from build123d import *

# Parameters (mm, degrees)
REVOLVE_3_ANGLE               = 210
SKETCH_11_W                   = 1123.766968822
SKETCH_11_H                   = 50
CUT_REVOLVE_6_ANGLE           = 5
CUT_REVOLVE_6_OTHER_WAY_ANGLE = 180


with BuildPart() as part:
    # 草图4 → 旋转3 (revolve)
    with BuildSketch(Plane.XY):
        Polygon((-949.526197638, 0), (-949.526197638, -80), (-700, -80), (-700, 80), (-949.526197638, 80), align=None)
    revolve(axis=Axis((0, 0, 0), (0, 1, 0)), revolution_arc=REVOLVE_3_ANGLE)

    # 草图10 → 切除-旋转5 (revolve, cut)
    with BuildSketch(Plane(origin=(0, 0, 0), x_dir=(0.9659258262890681, 0, -0.2588190451025215), z_dir=(0.2588190451025215, 0, 0.9659258262890681)), mode=Mode.PRIVATE) as cut_revolve_5_sk:
        with BuildLine():
            Line((-750, 50), (750, 50))
            ThreePointArc((750, 50), (785.355339059, 35.355339059), (800, 0))
            Line((800, 0), (-800, 0))
            ThreePointArc((-800, 0), (-785.355339059, 35.355339059), (-750, 50))
        make_face()
    revolve(cut_revolve_5_sk.sketch.rotate(Axis((-1280.947086283, 0, 343.228737317), (0.9659258262890681, 0, -0.25881904510252157)), 90), axis=Axis((-1280.947086283, 0, 343.228737317), (0.9659258262890681, 0, -0.25881904510252157)), mode=Mode.SUBTRACT)

    # 草图11 → 切除-旋转6 (revolve, cut)
    with BuildSketch(Plane(origin=(0, 0, 0), x_dir=(0.9659258262890681, 0, -0.2588190451025215), z_dir=(0.2588190451025215, 0, 0.9659258262890681))):
        with Locations((-561.883484411, 0)):
            Rectangle(SKETCH_11_W, SKETCH_11_H)
    revolve(axis=Axis((0, 25, 0), (0, -1, 0)), revolution_arc=CUT_REVOLVE_6_ANGLE, mode=Mode.SUBTRACT)

    # 草图11 → 切除-旋转6 other way (revolve, cut)
    with BuildSketch(Plane(origin=(0, 0, 0), x_dir=(0.9659258262890681, 0, -0.2588190451025215), z_dir=(0.2588190451025215, 0, 0.9659258262890681))):
        with Locations((-561.883484411, 0)):
            Rectangle(SKETCH_11_W, SKETCH_11_H)
    revolve(axis=Axis((0, 25, 0), (0, 1, 0)), revolution_arc=CUT_REVOLVE_6_OTHER_WAY_ANGLE, mode=Mode.SUBTRACT)


solid = part.part
Could you check a few things on this model? Use its own coordinates, in mm. A direction names the side the tool comes from. Round coordinates to 2 decimals unless told otherwise and drop trailing zeros. Write each loop counter-clockwise with the first axis right and the second up, starting at its lowest first coordinate (ties: lowest second). Pieces come first, ordered by that corner, then holes. Notation, with made-up numbers: (-5.75, -32) - (40.25, -32) arc R8 ccw to (40.25, -18) - close; hole circle Ø11 at (27.5, 27). An arc over 180 degrees is marked (long way). Use a Markdown table: item, result.
Q1. Please list where these lines run through material, in increasing order: L1, parallel to Y at x = -720, z = 618; L2, parallel to X at y = -29.5, z = 635; L3, parallel to X at y = 28.5, z = 299.
Output values:
| item | result |
|---|---|
| L1 | -80 to -25, 25 to 80 |
| L2 | -705.96 to -294.58, 294.58 to 705.96 |
| L3 | -901.22 to -632.93, 632.93 to 901.22 |
Q2. Thinking about a two-plate mould opening in X: for faces 1 (the cylindrical face through (-699.112, -49.995, 188.085)), 2 (the flat face through (49, -25, 710)), 3 (the flat face through (715.778, 1.12, -413.255)), 4 (the cylindrical face through (-699, 50, 187)), which applies, released by +X, released by -X, zero draft, split by the parting line, or undercut?
Output values:
| item | result |
|---|---|
| face 1 | undercut |
| face 2 | zero draft |
| face 3 | released by -X |
| face 4 | undercut |
Q3. I want a section at A-A (x = 0). List the corners of the cut face in (y, z) for me.
Output values:
| item | result |
|---|---|
| outline | (-80, 700) - (-25, 700) - (-25, 949.53) - (-80, 949.53) - close; (25, 700) - (80, 700) - (80, 949.53) - (25, 949.53) - close |
Q4. I want a section at B-B (z = 297.5). List the corners of the cut face in (x, y) for me, plus the area to 3 significant figures.
Output values:
| item | result |
|---|---|
| outline | (-901.72, -80) - (-633.64, -80) - (-633.64, -25) - (-901.72, -25) - close; (-901.72, 25) - (-633.64, 25) - (-633.64, 80) - (-901.72, 80) - close; (633.64, -80) - (901.72, -80) - (901.72, -25) - (633.64, -25) - close; (633.64, 25) - (901.72, 25) - (901.72, 80) - (633.64, 80) - close |
| area | 59,000 mm2 |
Q5. For pin 1 (2 mm diameter, centred on x = 226.5, y = 39, fed in from -Z); pin 2 (1 mm diameter, centred on x = 271, y = -57, fed in from -Z); pin 3 (12 mm diameter, centred on y = 40.5, z = 242, fed in from -X), each with a flat end and sliding along its axis, tell me the tip position at first contact or that it passes through.
Output values:
| item | result |
|---|---|
| pin 1 | z = 662 |
| pin 2 | z = 645.2 |
| pin 3 | x = -919.73 |
Q6. I want a section at C-C (x = 285.5). List the corners of the cut face in (y, z) for me, plus the area to 3 significant figures.
Output values:
| item | result |
|---|---|
| outline | (-80, 639.13) - (-25, 639.13) - (-25, 905.59) - (-80, 905.59) - close; (25, 639.13) - (80, 639.13) - (80, 905.59) - (25, 905.59) - close |
| area | 29,300 mm2 |
Q7. For faces 5 (the flat face through (842.777, 0.35, -225.822)), 6 (the flat face through (-827, 1, 0)), 7 (the cylindrical face through (222.146, -36.676, 923.175)), which set-ups out of +Z, -Z, +X, -X, +Y, -Y let a thin tool reach every point of the face, with its end or its side?
Output values:
| item | result |
|---|---|
| face 5 | +Z, +X |
| face 6 | -Z, -X, +Y, -Y |
| face 7 | +Y, -Y |
